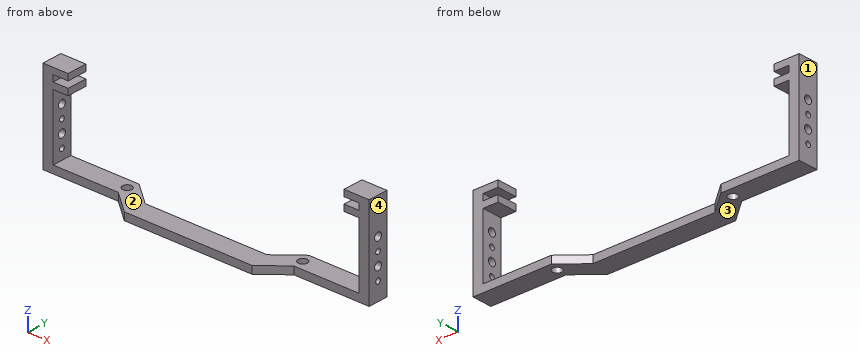
```python
from build123d import *

# Parameters (mm, degrees)
PAD_DEPTH         = 8
SKETCH002_R       = 1.85
POCKET_DEPTH      = 276.677278
POCKET_DEPTH_BACK = 302.677278
SKETCH_R          = 1.55
SKETCH_R_2        = 1.05
POCKET001_DEPTH   = 135.001


with BuildPart() as part:
    # Sketch001 → Pad (new body, symmetric)
    with BuildSketch(Plane.XZ):
        Polygon((-65, 36), (-65, 0), (0, 0), (0, 3), (-61, 3), (-61, 28.5), (-55, 28.5), (-55, 31), (-61, 31), (-61, 33.5), (-55, 33.5), (-55, 36), align=None)
    pad = extrude(amount=PAD_DEPTH, both=True)

    # Mirrored: Pad across Sketch001 V_Axis
    add(pad.mirror(Plane(origin=(0, 0, 0), x_dir=(0, -1, 0), z_dir=(1, 0, 0))))

    # Sketch002 → Pocket (cut, two sides)
    with BuildSketch(Plane.XY.offset(5)) as pocket_sk:
        with Locations((-35, 4)):
            Circle(SKETCH002_R)
        Polygon((-66, 0), (-35, 0), (-24.274218, -9), (-66, -9), align=None)
        Polygon((-35, 9), (-24.274218, 0), (0, 0), (0, 9), align=None)
    pocket = extrude(amount=-POCKET_DEPTH, mode=Mode.SUBTRACT) + extrude(pocket_sk.sketch, amount=POCKET_DEPTH_BACK, mode=Mode.SUBTRACT)

    # Mirrored001: Pocket across Sketch002 V_Axis
    add(pocket.mirror(Plane(origin=(0, 0, 5), x_dir=(0, 0, 1), z_dir=(1, 0, 0))), mode=Mode.SUBTRACT)

    # Sketch → Pocket001 (cut, through all)
    with BuildSketch(Plane.YZ.offset(70)):
        with Locations((4, 12)):
            Circle(SKETCH_R)
        with Locations((4, 7)):
            Circle(SKETCH_R_2)
        with Locations((4, 17)):
            Circle(SKETCH_R_2)
        with Locations((4, 22)):
            Circle(SKETCH_R)
    extrude(amount=-POCKET001_DEPTH, mode=Mode.SUBTRACT)


solid = part.part
```
Work out the finished part from the listing and answer in its coordinate system (mm). Face numbers are marked on the shaded views. Give positions to 0.01 mm unless a question says otherwise; leave off trailing zeros. Write each loop counter-clockwise with the first axis right and the second up, starting at its lowest first coordinate (ties: lowest second). Pieces come first, ordered by that corner, then holes. Notation, with made-up numbers: (39, -35) -> (48, -35) arc R22 cw to (48, 2) -> close; hole circle Ø8 at (-20, 9). An arc over 180 degrees is marked (long way). Write item = value, one per line.
Q1. Section B-B on y = -5.25 is taken. Determine the outline of the cut face in (x, z), and give its area (3 significant figures).
Computed values:
outline = (-28.74, 0) -> (28.74, 0) -> (28.74, 3) -> (-28.74, 3) -> close
area = 172 mm^2
Q2. Flat-ended cylindrical pins translate along their axes: pin 1 Ø5 at (x, y) = (57, 6) entering from -Z; pin 2 Ø2.5 at (y, z) = (4, 12) entering from -X; pin 3 Ø1.5 at (x, z) = (-9.5, 2) entering from +Y; pin 4 Ø8 at (x, y) = (47, 1) entering from +Z. Find the tip coordinate at first contact, or state that the pin passes through.
Computed values:
pin_1 = 0
pin_2 = through
pin_3 = 0
pin_4 = 3
Q3. Section A-A on x = 3 is taken. Determine the outline of the cut face in (y, z), and give its area (3 significant figures).
Computed values:
outline = (-8, 0) -> (0, 0) -> (0, 3) -> (-8, 3) -> close
area = 24.0 mm^2
Q4. For a pull along X with two mould halves and no side action, classify the marked faces 1, 2, 3 and 4 as pulls with the +X half, pulls with the -X half, needs draft (parallel to the pull), parting line crosses it, or undercut.
Computed values:
face_1 = pulls with the -X half
face_2 = undercut
face_3 = needs draft
face_4 = pulls with the +X half
Q5. Consider line 1 along Z through (x, y) = (-62.15, 4); line 2 along Z through (x, y) = (55.5, 5.5); line 3 along X through (y, z) = (5.25, 24). Determine where each line is inside the solid, lowest interval first.
Computed values:
line_1 = 0 to 5.95, 8.05 to 10.45, 13.55 to 15.95, 18.05 to 20.45, 23.55 to 36
line_2 = 0 to 3, 28.5 to 31, 33.5 to 36
line_3 = -65 to -61, 61 to 65
